Here's how the part is built. I have some questions about the finished solid (model axes, mm). Round coordinates to 2 decimals unless told otherwise and drop trailing zeros. Answer in a Markdown table with one row per item.
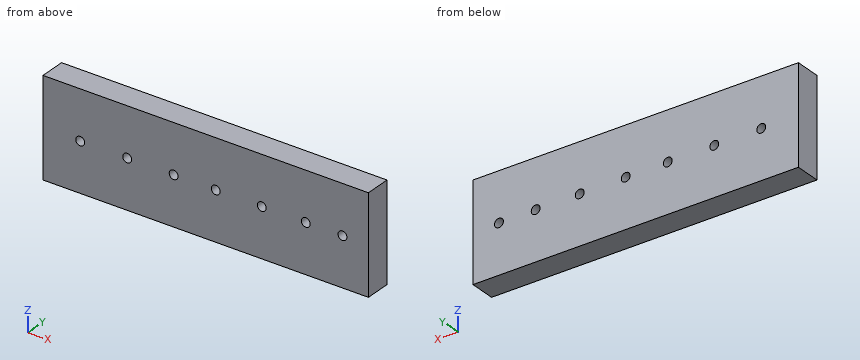
```python
from build123d import *

# Parameters (mm, degrees)
F0_W     = 127
F0_H     = 38.1
F1_DEPTH = 10
F3_D     = 3.44678
F4_D     = 3.44932
F5_D     = 3.45186
F6_D     = 3.4544
F7_D     = 3.45694
F8_D     = 3.45948
F9_D     = 3.46202


with BuildPart() as f1:
    # F0 (on Front) → F1 (new body)
    with BuildSketch(Plane.XZ):
        with Locations((63.5, -19.05)):
            Rectangle(F0_W, F0_H)
    extrude(amount=F1_DEPTH)

    # F3 (through all)
    with Locations(Plane(origin=(0, 0, 0), x_dir=(1, 0, 0), z_dir=(0, 1, 0))):
        with Locations((14.5125538111, 19.05)):
            Hole(F3_D / 2)

    # F4 (through all)
    with Locations(Plane(origin=(0, 0, 0), x_dir=(1, 0, 0), z_dir=(0, 1, 0))):
        with Locations((32.8442007303, 19.05)):
            Hole(F4_D / 2)

    # F5 (through all)
    with Locations(Plane(origin=(0, 0, 0), x_dir=(1, 0, 0), z_dir=(0, 1, 0))):
        with Locations((85.3567272425, 19.05)):
            Hole(F5_D / 2)

    # F6 (through all)
    with Locations(Plane(origin=(0, 0, 0), x_dir=(1, 0, 0), z_dir=(0, 1, 0))):
        with Locations((116.8642491102, 19.05)):
            Hole(F6_D / 2)

    # F7 (through all)
    with Locations(Plane(origin=(0, 0, 0), x_dir=(1, 0, 0), z_dir=(0, 1, 0))):
        with Locations((50.9848929942, 19.05)):
            Hole(F7_D / 2)

    # F8 (through all)
    with Locations(Plane(origin=(0, 0, 0), x_dir=(1, 0, 0), z_dir=(0, 1, 0))):
        with Locations((67.4069970846, 19.05)):
            Hole(F8_D / 2)

    # F9 (through all)
    with Locations(Plane(origin=(0, 0, 0), x_dir=(1, 0, 0), z_dir=(0, 1, 0))):
        with Locations((102.5426462293, 19.05)):
            Hole(F9_D / 2)


solid = f1.part
```
1. For pin 1 Ø4 at (x, z) = (45, -24.5) entering from +Y, with a flat end and sliding along its axis, tell me the tip position at first contact or that it passes through.
Numbers:
| item | result |
|---|---|
| pin 1 | stops at y = 0 |
2. Suppose I cut it at A-A on z = -19.05. State how many separate pieces and enclosed holes the cut face has, then the cut area to 3 significant figures.
Numbers:
| item | result |
|---|---|
| separate pieces | 8 |
| enclosed holes | 0 |
| area | 1,030 mm2 |
3. Please list where this line runs through material, in increasing order: line 1 along Z through (x, y) = (13.5, -6.75).
Numbers:
| item | result |
|---|---|
| line 1 | z = -38.1 to -20.44, -17.66 to 0 |
